```python
from build123d import *

# Parameters (mm, degrees)
SKETCH1_R           = 25
SKETCH1_R_2         = 22
BOSS_EXTRUDE1_DEPTH = 100
SKETCH2_W           = 10
SKETCH2_H           = 10
BOSS_EXTRUDE3_DEPTH = 3
FILLET2_R           = 3
FILLET3_R           = 3
SKETCH3_W           = 4
SKETCH3_H           = 10
BOSS_EXTRUDE4_DEPTH = 12
CUT_EXTRUDE1_REACH  = 111.309
SKETCH4_R           = 1.5
FILLET4_R           = 3
SKETCH5_W           = 63.273881994
SKETCH5_H           = 26.217893921
CUT_EXTRUDE2_DEPTH  = 50
BOSS_EXTRUDE5_DEPTH = 50


with BuildPart() as part:
    # Sketch1 → Boss-Extrude1 (new body)
    with BuildSketch(Plane.XY):
        Circle(SKETCH1_R)
        Circle(SKETCH1_R_2, mode=Mode.SUBTRACT)
    extrude(amount=BOSS_EXTRUDE1_DEPTH)

    # Sketch2 → Boss-Extrude3 (add)
    with BuildSketch(Plane(origin=(0, 0, 0), x_dir=(-1, 0, 0), z_dir=(0, 0, -1))):
        with Locations((0, 19.494897428)):
            Rectangle(SKETCH2_W, SKETCH2_H)
    extrude(amount=-BOSS_EXTRUDE3_DEPTH)

    # Fillet2
    # the kernel refuses this fillet: 3 mm, written as the material it adds along each edge
    with BuildSketch(Plane(origin=(0, 0, 3), x_dir=(-0.5397978604012739, 0.8417946720585768, 0), z_dir=(-0.8417946720585768, -0.5397978604012739, 0))) as fillet2_piece_1_section:
        with BuildLine():
            CenterArc((22 - FILLET2_R, -FILLET2_R), FILLET2_R, 0, 90)
            Line((22 - FILLET2_R, 0), (22, 0))
            Line((22, 0), (22, -FILLET2_R))
        make_face()
    fillet2_piece_1 = revolve(axis=Axis((0, 0, 3), (0, 0, -1)), revolution_arc=65.339758778, mode=Mode.PRIVATE)
    fillet2_piece_1 = split(fillet2_piece_1, bisect_by=Plane(origin=(5, 21.121644808, 3.678956026), z_dir=(-1, 0, 0)), keep=Keep.TOP, mode=Mode.PRIVATE)
    fillet2_piece_1 = split(fillet2_piece_1, bisect_by=Plane(origin=(-5, 21.121644808, 3.678956026), z_dir=(1, 0, 0)), keep=Keep.TOP, mode=Mode.PRIVATE)
    add(fillet2_piece_1)
    with BuildSketch(Plane(origin=(5, 21.424285286, 3), x_dir=(0.9454116384931546, -0.32587855683013084, 0), z_dir=(0, 0, -1))) as fillet2_piece_2:
        with BuildLine():
            CenterArc((4.201860731, 2.984203833), FILLET2_R, 160.981189421, 114.90106237)
            Line((1.365625815, 3.961839503), (0, 0))
            ThreePointArc((0, 0), (2.254656978, -0.11583856), (4.509313955, 0))
        make_face()
    extrude(amount=3)
    with BuildSketch(Plane(origin=(-5, 21.424285286, 3), x_dir=(-0.9454116384931545, -0.325878556830131, 0), z_dir=(0, 0, -1))) as fillet2_piece_3:
        with BuildLine():
            CenterArc((4.201860731, -2.984203833), FILLET2_R, 84.117748208, 114.90106237)
            Line((1.365625815, -3.961839503), (0, 0))
            ThreePointArc((0, 0), (2.254656978, 0.11583856), (4.509313955, 0))
        make_face()
    extrude(amount=3)
    with BuildSketch(Plane(origin=(0, 0, 3), x_dir=(-0.5397978604012739, 0.8417946720585768, 0), z_dir=(-0.8417946720585768, -0.5397978604012739, 0))) as fillet2_piece_4a_section:
        with BuildLine():
            CenterArc((22 - FILLET2_R, -FILLET2_R), FILLET2_R, 0, 90)
            Line((22 - FILLET2_R, 0), (22, 0))
            Line((22, 0), (22, -FILLET2_R))
        make_face()
    fillet2_piece_4a = revolve(axis=Axis((0, 0, 3), (0, 0, -1)), revolution_arc=65.339758778, mode=Mode.PRIVATE)
    fillet2_piece_4a = split(fillet2_piece_4a, bisect_by=Plane(origin=(-5, 19.550370475, 3.699165733), z_dir=(-1, 0, 0)), keep=Keep.TOP, mode=Mode.PRIVATE)
    with BuildSketch(Plane(origin=(-5, 21.424285286, 14.273284888), x_dir=(-0.9454116384931546, -0.3258785568301304, 0), z_dir=(0, 0, -1))) as fillet2_piece_4b_section:
        with BuildLine():
            CenterArc((4.201860731, -2.984203833), FILLET2_R, 84.117748208, 114.90106237)
            Line((1.365625815, -3.961839503), (0, 0))
            ThreePointArc((0, 0), (2.254656978, 0.11583856), (4.509313955, 0))
        make_face()
    fillet2_piece_4b = extrude(amount=14.273284888, mode=Mode.PRIVATE)
    fillet2_piece_4b = split(fillet2_piece_4b, bisect_by=Plane(origin=(-6.027024326, 20.156097629, 3), z_dir=(0, 0, 1)), keep=Keep.TOP, mode=Mode.PRIVATE)
    fillet2_piece_4 = fillet2_piece_4a & fillet2_piece_4b
    add(fillet2_piece_4)
    with BuildSketch(Plane(origin=(5, 21.424285286, 14.273284888), x_dir=(0.9454116384931546, -0.32587855683013073, 0), z_dir=(0, 0, -1))) as fillet2_piece_5a_section:
        with BuildLine():
            CenterArc((4.201860731, 2.984203833), FILLET2_R, 160.981189421, 114.90106237)
            Line((1.365625815, 3.961839503), (0, 0))
            ThreePointArc((0, 0), (2.254656978, -0.11583856), (4.509313955, 0))
        make_face()
    fillet2_piece_5a = extrude(amount=14.273284888, mode=Mode.PRIVATE)
    fillet2_piece_5a = split(fillet2_piece_5a, bisect_by=Plane(origin=(6.027024326, 20.156097629, 3), z_dir=(0, 0, 1)), keep=Keep.TOP, mode=Mode.PRIVATE)
    with BuildSketch(Plane(origin=(0, 0, 3), x_dir=(-0.5397978604012739, 0.8417946720585768, 0), z_dir=(-0.8417946720585768, -0.5397978604012739, 0))) as fillet2_piece_5b_section:
        with BuildLine():
            CenterArc((22 - FILLET2_R, -FILLET2_R), FILLET2_R, 0, 90)
            Line((22 - FILLET2_R, 0), (22, 0))
            Line((22, 0), (22, -FILLET2_R))
        make_face()
    fillet2_piece_5b = revolve(axis=Axis((0, 0, 3), (0, 0, -1)), revolution_arc=65.339758778, mode=Mode.PRIVATE)
    fillet2_piece_5b = split(fillet2_piece_5b, bisect_by=Plane(origin=(5, 19.550370668, 3.699165846), z_dir=(1, 0, 0)), keep=Keep.TOP, mode=Mode.PRIVATE)
    fillet2_piece_5 = fillet2_piece_5a & fillet2_piece_5b
    add(fillet2_piece_5)

    # Fillet3
    fillet3_edges = [part.edges().sort_by_distance(p)[0] for p in [
        (-5, 14.494897428, 1.5),
        (5, 14.494897428, 1.5),
    ]]
    fillet(fillet3_edges, radius=FILLET3_R)

    # Sketch3 → Boss-Extrude4 (add)
    with BuildSketch(Plane(origin=(0, 0, 0), x_dir=(-1, 0, 0), z_dir=(0, 0, -1))):
        with Locations((0, -29.919871589)):
            Rectangle(SKETCH3_W, SKETCH3_H)
    extrude(amount=-BOSS_EXTRUDE4_DEPTH)

    # Sketch4 → Cut-Extrude1 (cut, up to next)
    with BuildSketch(Plane.ZY.offset(2), mode=Mode.PRIVATE) as cut_extrude1_sk1:
        with Locations(Location((5, -30.919871589, 0), (0, 0, 270))):
            Circle(SKETCH4_R)
    cut_extrude1_tool1 = extrude(cut_extrude1_sk1.sketch, amount=-CUT_EXTRUDE1_REACH, mode=Mode.PRIVATE) & part.part
    add(cut_extrude1_tool1.solids().sort_by_distance((-2, -30.919872, 5))[0], mode=Mode.SUBTRACT)

    # Fillet4
    fillet4_edges = [part.edges().sort_by_distance(p)[0] for p in [
        (0, -25, 12),
        (-2, -24.919871589, 6),
        (0, -34.919871589, 12),
        (2, -24.919871589, 6),
        (0, -34.919871589, 0),
    ]]
    fillet(fillet4_edges, radius=FILLET4_R)

    # Sketch5 → Cut-Extrude2 (cut)
    with BuildSketch(Plane.XY.offset(100)):
        with Locations((0, 13.108946961)):
            Rectangle(SKETCH5_W, SKETCH5_H)
    extrude(amount=-CUT_EXTRUDE2_DEPTH, mode=Mode.SUBTRACT)

    # Sketch8 → Boss-Extrude5 (add)
    with BuildSketch(Plane.XY.offset(100)):
        Polygon((25, 0), (22, 0), (32.606601718, 10.606601718), (34.106601718, 9.106601718), align=None)
        Polygon((-25, 0), (-22, 0), (-32.606601718, 10.606601718), (-34.106601718, 9.106601718), align=None)
    extrude(amount=-BOSS_EXTRUDE5_DEPTH)


solid = part.part
```
The listing builds one solid part. Answer for the finished solid, in the listing's coordinates (mm). A direction names the side the tool comes from. Coordinates: 2 decimals unless noted, no trailing zeros. Write each loop counter-clockwise with the first axis right and the second up, starting at its lowest first coordinate (ties: lowest second). Pieces come first, ordered by that corner, then holes. Notation, with made-up numbers: (-28.5, 46) - (-18.5, 46) arc R19 cw to (-18.5, 60) - close; hole circle Ø6 at (63, -1). An arc over 180 degrees is marked (long way). One line per item, written item: value.
1) Each of these flat-tipped pins is pushed along its axis until it touches: pin 1 Ø4 at (y, z) = (3.5, 35.5) entering from +X; pin 2 Ø1 at (x, z) = (12, 46.5) entering from -Y; pin 3 Ø5 at (x, y) = (1.5, 17) entering from +Z; pin 4 Ø4 at (x, y) = (25, -11.5) entering from +Z. Where does it stop, or does it pass through?
Geometry check:
pin 1: stops at x = 24.95
pin 2: stops at y = -22.2
pin 3: stops at z = 3.05
pin 4: passes through
2) Find section A-A (x = 0). Give the vertices of the cut face in (y, z).
Geometry check:
outline: (-34.92, 3) arc R3 ccw to (-31.92, 0) - (-22, 0) - (-22, 100) - (-25, 100) - (-25, 15) arc R3 cw to (-28, 12) - (-31.92, 12) arc R3 ccw to (-34.92, 9) - close; (14.49, 0) - (25, 0) - (25, 50) - (22, 50) - (22, 6) arc R3 cw to (19, 3) - (14.49, 3) - close; hole circle Ø3 at (-30.92, 5)
3) Find section D-D (x = -11.5). Give the vertices of the cut face in (y, z) (3 decimals).
Geometry check:
outline: (-22.198, 0) - (-18.755, 0) - (-18.755, 100) - (-22.198, 100) - close; (18.755, 0) - (22.198, 0) - (22.198, 50) - (18.755, 50) - close
4) A tool of negligible diameter and unlimited length cuts with its end or side. For faces 1 (the cylindrical face through (6.99, 20.06, 2.38)), 2 (the flat face through (-27, 5, 75)), 3 (the flat face through (-2, -31, 7)), from which of +Z, -Z, +X, -X, +Y, -Y can it reach the whole face along a straight path? Write none if from no direction.
Geometry check:
face 1: +Z, -Z
face 2: +Z, +Y
face 3: +Z, -Z, -X, -Y
5) Find section B-B (z = 62). Give the vertices of the cut face in (x, y).
Geometry check:
outline: (-34.11, 9.11) - (-25, 0) arc R25 ccw to (25, 0) - (34.11, 9.11) - (32.61, 10.61) - (22, 0) arc R22 cw to (-22, 0) - (-32.61, 10.61) - close
6) Find section C-C (y = -3.5). Give the vertices of the cut face in (x, z), and give its area (3 significant figures).
Geometry check:
outline: (-24.75, 0) - (-21.72, 0) - (-21.72, 100) - (-24.75, 100) - close; (21.72, 0) - (24.75, 0) - (24.75, 100) - (21.72, 100) - close
area: 607 mm2
7) For a pull along Y with two mould halves and no side action, classify faces 4 (the cylindrical face through (11.5, -22.2, 38.2)), 5 (the flat face through (0, -30, 12)), 6 (the flat face through (30, 5, 75)), 7 (the flat face through (0, 17, 3)) as pulls with the +Y half, pulls with the -Y half, needs draft (parallel to the pull), parting line crosses it, or undercut.
Geometry check:
face 4: parting line crosses it
face 5: needs draft
face 6: pulls with the -Y half
face 7: undercut
8) Consider line 1 along Y through (x, z) = (0, 32); line 2 along Z through (x, y) = (-3, 22). Determine where each line is inside the solid, lowest interval first. Write a range as from..to.
Geometry check:
line 1: y = -25..-22, 22..25
line 2: z = 0..50
